Could you check a few things on this drawing? It's one solid part, dimensions in mm from its lowest x, y, z. A direction names the side the tool comes from. Round coordinates to 2 decimals unless told otherwise and drop trailing zeros. Loops run counter-clockwise (first coordinate to the right, second up) from the corner with the lowest first, then second, coordinate; pieces in that order, holes last. Notation, with made-up numbers: M 54.25,68 L 61.25,68 A22 cw 61.25,106 Z; hole C 43,27.5 d6. An arc over 180 degrees is marked long. Write item = value, one per line. Start each with the question number.
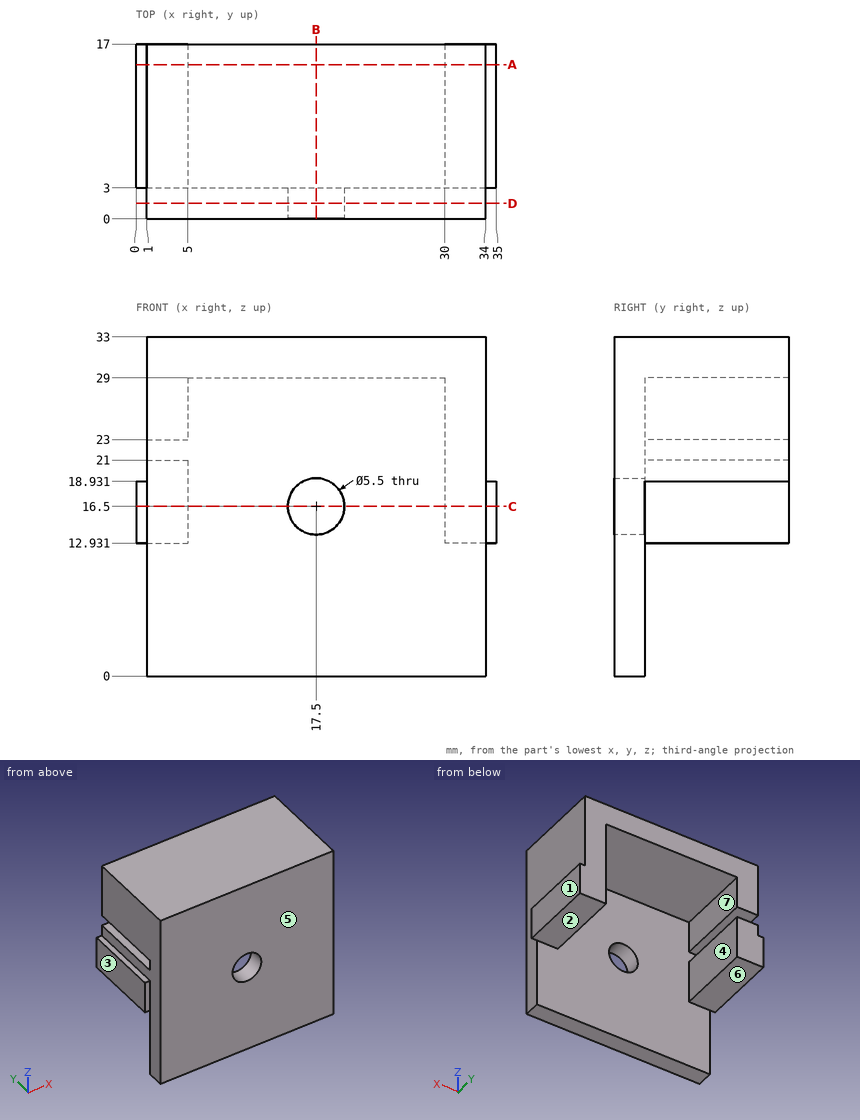
Item 1: I want a section at A-A, the plane y = 15. List the corners of the cut face in (x, z) for me.
Item 2: I want a section at D-D, the plane y = 1.5. List the corners of the cut face in (x, z) for me.
Item 3: Will these pins go through, and if not, where does the flat tip stop? pin 1 Ø1 at (x, z) = (12, 15.5) entering from +Y; pin 2 Ø0.5 at (x, y) = (34.5, 11.5) entering from +Z; pin 3 Ø1 at (x, z) = (22, 23) entering from -Y; pin 4 Ø7 at (x, y) = (19.5, 10) entering from -Z.
Item 4: Please list where these lines run through material, in increasing order: line 1 (Z direction, x = 17.5, y = 1.7); line 2 (X direction, y = 2.2, z = 16.5); line 3 (X direction, y = 13, z = 27). Write a range as [from, to].
Item 5: We'd pull the mould along X, two halves only. Please class the marked faces 1, 2, 3 and 4: released by +X, released by -X, zero draft, split by the parting line, or undercut.
Item 6: I want a section at B-B, the plane x = 17.5. List the corners of the cut face in (y, z) for me.
Item 7: I want a section at C-C, the plane z = 16.5. List the corners of the cut face in (x, y) for me.
Item 8: For the marked faces 5, 6 and 7, which set-ups out of +Z, -Z, +X, -X, +Y, -Y let a thin tool reach every point of the face, with its end or its side?
Worked out:
q1.outline = M 0,12.93 L 5,12.93 L 5,21 L 1,21 L 1,18.93 L 0,18.93 Z; M 1,23 L 5,23 L 5,29 L 30,29 L 30,12.93 L 35,12.93 L 35,18.93 L 34,18.93 L 34,33 L 1,33 Z
q2.outline = M 1,0 L 34,0 L 34,33 L 1,33 Z; hole C 17.5,16.5 d5.5
q3.pin_1 = 3
q3.pin_2 = 18.93
q3.pin_3 = 0
q3.pin_4 = 29
q4.line_1 = [0, 13.75], [19.25, 33]
q4.line_2 = [1, 14.75], [20.25, 34]
q4.line_3 = [1, 5], [30, 34]
q5.face_1 = released by +X
q5.face_2 = zero draft
q5.face_3 = released by -X
q5.face_4 = undercut
q6.outline = M 0,0 L 3,0 L 3,13.75 L 0,13.75 Z; M 0,19.25 L 3,19.25 L 3,29 L 17,29 L 17,33 L 0,33 Z
q7.outline = M 0,3 L 1,3 L 1,0 L 14.75,0 L 14.75,3 L 5,3 L 5,17 L 0,17 Z; M 20.25,0 L 34,0 L 34,3 L 35,3 L 35,17 L 30,17 L 30,3 L 20.25,3 Z
q8.face_5 = +Z, -Z, +X, -X, -Y
q8.face_6 = -Z, +X, -X, +Y
q8.face_7 = -Z, +Y
